```python
from build123d import *

# Parameters (mm, degrees)
SKETCH2_W           = 90
SKETCH2_H           = 42.5
SKETCH2_R           = 11
SKETCH2_R_2         = 1.6
SKETCH2_R_3         = 4.79806
BOSS_EXTRUDE1_DEPTH = 3.175


with BuildPart() as part:
    # Sketch2 → Boss-Extrude1 (new body)
    with BuildSketch(Plane(origin=(0, 0, 0), x_dir=(1, 0, 0), z_dir=(0, 1, 0))):
        Rectangle(SKETCH2_W, SKETCH2_H)
        Circle(SKETCH2_R, mode=Mode.SUBTRACT)
        with Locations((-15.5, 15.5)):
            Circle(SKETCH2_R_2, mode=Mode.SUBTRACT)
        with Locations((15.5, 15.5)):
            Circle(SKETCH2_R_2, mode=Mode.SUBTRACT)
        with Locations((15.5, -15.5)):
            Circle(SKETCH2_R_2, mode=Mode.SUBTRACT)
        with Locations((-15.5, -15.5)):
            Circle(SKETCH2_R_2, mode=Mode.SUBTRACT)
        with Locations((-37.5, 0)):
            Circle(SKETCH2_R_3, mode=Mode.SUBTRACT)
        with Locations((37.5, 0)):
            Circle(SKETCH2_R_3, mode=Mode.SUBTRACT)
    extrude(amount=BOSS_EXTRUDE1_DEPTH)


solid = part.part
```
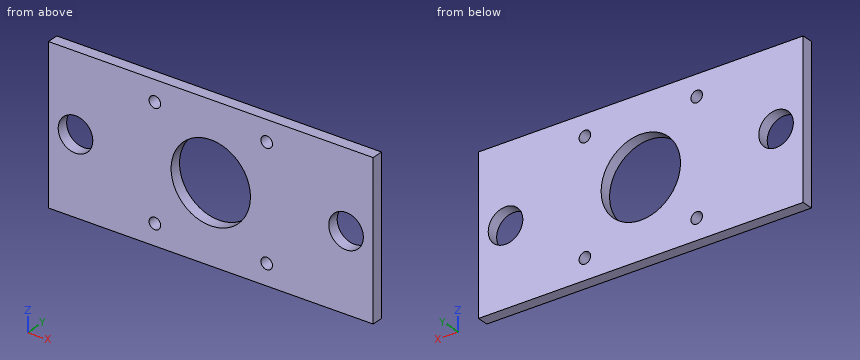
Can you work these out from the model? Positions are in its coordinate system, mm. Round coordinates to 2 decimals unless told otherwise and drop trailing zeros. Order: outer loops, then holes, each group sorted by start corner. A loop starts at its lowest first (then second) coordinate and runs counter-clockwise, first axis right, second up. Notation, with made-up numbers: (28.25, 88) -> (64.25, 88) arc R13 cw to (64.25, 104) -> close; hole circle Ø8 at (69.25, 57). An arc over 180 degrees is marked (long way). Return JSON: item names as keys, results as strings. Group by question number.
1. Will this pin go through, and if not, where does the flat tip stop? pin 1 (7.5 mm diameter, centred on x = 37.5, z = 0, fed in from +Y).
2. I need wall thicknesses on line 1 (X direction, y = 1.3, z = -15.5); line 2 (X direction, y = 1.7, z = 0); line 3 (Z direction, x = 15.5, y = 1.9). Which ranges of each line are inside material? Lowest first, please. Write a range as [from, to].
3. If we section it at D-D, the plane x = 0: Write out the boundary of the cut face in (y, z) (3 decimals).
4. If we section it at B-B, the plane z = -15.5: Write out the boundary of the cut face in (x, y) (3 decimals), then the cut area to 3 significant figures.
5. If we section it at A-A, the plane x = -15.5: Write out the boundary of the cut face in (y, z) (3 decimals).
6. If we section it at C-C, the plane y = 0.7: Write out the boundary of the cut face in (x, z).
Output values:
{
 "1": {"pin 1": "through"},
 "2": {"line 1": "[-45, -17.1], [-13.9, 13.9], [17.1, 45]", "line 2": "[-45, -42.3], [-32.7, -11], [11, 32.7], [42.3, 45]", "line 3": "[-21.25, -17.1], [-13.9, 13.9], [17.1, 21.25]"},
 "3": {"outline": "(0, -21.25) -> (3.175, -21.25) -> (3.175, -11) -> (0, -11) -> close; (0, 11) -> (3.175, 11) -> (3.175, 21.25) -> (0, 21.25) -> close"},
 "4": {"outline": "(-45, 0) -> (-17.1, 0) -> (-17.1, 3.175) -> (-45, 3.175) -> close; (-13.9, 0) -> (13.9, 0) -> (13.9, 3.175) -> (-13.9, 3.175) -> close; (17.1, 0) -> (45, 0) -> (45, 3.175) -> (17.1, 3.175) -> close", "area": "265 mm²"},
 "5": {"outline": "(0, -21.25) -> (3.175, -21.25) -> (3.175, -17.1) -> (0, -17.1) -> close; (0, -13.9) -> (3.175, -13.9) -> (3.175, 13.9) -> (0, 13.9) -> close; (0, 17.1) -> (3.175, 17.1) -> (3.175, 21.25) -> (0, 21.25) -> close"},
 "6": {"outline": "(-45, -21.25) -> (45, -21.25) -> (45, 21.25) -> (-45, 21.25) -> close; hole circle Ø9.6 at (-37.5, 0); hole circle Ø3.2 at (-15.5, -15.5); hole circle Ø3.2 at (-15.5, 15.5); hole circle Ø22 at (0, 0); hole circle Ø3.2 at (15.5, -15.5); hole circle Ø3.2 at (15.5, 15.5); hole circle Ø9.6 at (37.5, 0)"}
}
